```python
from build123d import *

# Parameters (mm, degrees)
SKETCH1_W           = 96
SKETCH1_H           = 24.5
BOSS_EXTRUDE1_DEPTH = 3
BOSS_EXTRUDE2_DEPTH = 57
FILLET1_R           = 2
FILLET2_R           = 3
CUT_EXTRUDE1_REACH  = 117.231
CUT_EXTRUDE2_REACH  = 116.303
SKETCH5_W           = 16
SKETCH5_H           = 12
SKETCH5_W_2         = 24
BOSS_EXTRUDE3_DEPTH = 9
SKETCH6_W           = 2.75
SKETCH6_H           = 4
CUT_EXTRUDE3_DEPTH  = 6
LPATTERN1_COUNT     = 4
LPATTERN1_PITCH     = 3.75
SKETCH7_W           = 2.75
SKETCH7_H           = 4
CUT_EXTRUDE4_DEPTH  = 6
LPATTERN2_COUNT     = 6
LPATTERN2_PITCH     = 3.75


with BuildPart() as part:
    # Sketch1 → Boss-Extrude1 (new body)
    with BuildSketch(Plane(origin=(0, 0, 0), x_dir=(1, 0, 0), z_dir=(0, 1, 0))):
        with Locations((48, 12.25)):
            Rectangle(SKETCH1_W, SKETCH1_H)
    extrude(amount=BOSS_EXTRUDE1_DEPTH)

    # Sketch2 → Boss-Extrude2 (add)
    with BuildSketch(Plane(origin=(0, 3, 0), x_dir=(1, 0, 0), z_dir=(0, 1, 0))):
        Polygon((0, 0), (96, 0), (96, 3), (89, 3), (89, 24.5), (7, 24.5), (7, 3), (0, 3), align=None)
    extrude(amount=BOSS_EXTRUDE2_DEPTH)

    # Fillet1
    fillet1_edges = [part.edges().sort_by_distance(p)[0] for p in [
        (89, 31.5, -24.5),
        (7, 31.5, -24.5),
        (48, 60, -24.5),
    ]]
    fillet(fillet1_edges, radius=FILLET1_R)

    # Fillet2
    fillet2_edges = [part.edges().sort_by_distance(p)[0] for p in [
        (0, 60, -1.5),
        (96, 60, -1.5),
        (0, 1.5, -24.5),
        (96, 1.5, -24.5),
    ]]
    fillet(fillet2_edges, radius=FILLET2_R)

    # Sketch3 → Cut-Extrude1 (cut, up to next)
    with BuildSketch(Plane(origin=(0, 0, -3), x_dir=(-1, 0, 0), z_dir=(0, 0, -1)), mode=Mode.PRIVATE) as cut_extrude1_sk1:
        with BuildLine():
            Line((-93, 45.5), (-96, 45.5))
            Line((-96, 45.5), (-96, 40.5))
            Line((-96, 40.5), (-93, 40.5))
            ThreePointArc((-93, 40.5), (-90.5, 43), (-93, 45.5))
        make_face()
    cut_extrude1_tool1 = extrude(cut_extrude1_sk1.sketch, amount=-CUT_EXTRUDE1_REACH, mode=Mode.PRIVATE) & part.part
    # Sketch3 → Cut-Extrude1 (cut, up to next)
    with BuildSketch(Plane(origin=(0, 0, -3), x_dir=(-1, 0, 0), z_dir=(0, 0, -1)), mode=Mode.PRIVATE) as cut_extrude1_sk2:
        with BuildLine():
            Line((-93, 25.5), (-96, 25.5))
            Line((-96, 25.5), (-96, 20.5))
            Line((-96, 20.5), (-93, 20.5))
            ThreePointArc((-93, 20.5), (-90.5, 23), (-93, 25.5))
        make_face()
    cut_extrude1_tool2 = extrude(cut_extrude1_sk2.sketch, amount=-CUT_EXTRUDE1_REACH, mode=Mode.PRIVATE) & part.part
    # Sketch3 → Cut-Extrude1 (cut, up to next)
    with BuildSketch(Plane(origin=(0, 0, -3), x_dir=(-1, 0, 0), z_dir=(0, 0, -1)), mode=Mode.PRIVATE) as cut_extrude1_sk3:
        with BuildLine():
            Line((-3, 25.5), (0, 25.5))
            Line((0, 25.5), (0, 20.5))
            Line((0, 20.5), (-3, 20.5))
            ThreePointArc((-3, 20.5), (-5.5, 23), (-3, 25.5))
        make_face()
    cut_extrude1_tool3 = extrude(cut_extrude1_sk3.sketch, amount=-CUT_EXTRUDE1_REACH, mode=Mode.PRIVATE) & part.part
    # Sketch3 → Cut-Extrude1 (cut, up to next)
    with BuildSketch(Plane(origin=(0, 0, -3), x_dir=(-1, 0, 0), z_dir=(0, 0, -1)), mode=Mode.PRIVATE) as cut_extrude1_sk4:
        with BuildLine():
            Line((-3, 45.5), (0, 45.5))
            Line((0, 45.5), (0, 40.5))
            Line((0, 40.5), (-3, 40.5))
            ThreePointArc((-3, 40.5), (-5.5, 43), (-3, 45.5))
        make_face()
    cut_extrude1_tool4 = extrude(cut_extrude1_sk4.sketch, amount=-CUT_EXTRUDE1_REACH, mode=Mode.PRIVATE) & part.part
    add(cut_extrude1_tool1.solids().sort_by_distance((93.486888, 43, -3))[0], mode=Mode.SUBTRACT)
    add(cut_extrude1_tool2.solids().sort_by_distance((93.486888, 23, -3))[0], mode=Mode.SUBTRACT)
    add(cut_extrude1_tool3.solids().sort_by_distance((2.513112, 23, -3))[0], mode=Mode.SUBTRACT)
    add(cut_extrude1_tool4.solids().sort_by_distance((2.513112, 43, -3))[0], mode=Mode.SUBTRACT)

    # Sketch4 → Cut-Extrude2 (cut, up to next)
    with BuildSketch(Plane(origin=(0, 3, 0), x_dir=(1, 0, 0), z_dir=(0, 1, 0)), mode=Mode.PRIVATE) as cut_extrude2_sk1:
        with BuildLine():
            Line((3, 16.5), (0, 16.5))
            Line((0, 16.5), (0, 11.5))
            Line((0, 11.5), (3, 11.5))
            ThreePointArc((3, 11.5), (5.5, 14), (3, 16.5))
        make_face()
    cut_extrude2_tool1 = extrude(cut_extrude2_sk1.sketch, amount=-CUT_EXTRUDE2_REACH, mode=Mode.PRIVATE) & part.part
    # Sketch4 → Cut-Extrude2 (cut, up to next)
    with BuildSketch(Plane(origin=(0, 3, 0), x_dir=(1, 0, 0), z_dir=(0, 1, 0)), mode=Mode.PRIVATE) as cut_extrude2_sk2:
        with BuildLine():
            Line((93, 11.5), (96, 11.5))
            Line((96, 11.5), (96, 16.5))
            Line((96, 16.5), (93, 16.5))
            ThreePointArc((93, 16.5), (90.5, 14), (93, 11.5))
        make_face()
    cut_extrude2_tool2 = extrude(cut_extrude2_sk2.sketch, amount=-CUT_EXTRUDE2_REACH, mode=Mode.PRIVATE) & part.part
    add(cut_extrude2_tool1.solids().sort_by_distance((2.513112, 3, -14))[0], mode=Mode.SUBTRACT)
    add(cut_extrude2_tool2.solids().sort_by_distance((93.486888, 3, -14))[0], mode=Mode.SUBTRACT)

    # Sketch5 → Boss-Extrude3 (add)
    with BuildSketch(Plane(origin=(0, 60, 0), x_dir=(1, 0, 0), z_dir=(0, 1, 0))):
        with Locations((68.5, 12)):
            Rectangle(SKETCH5_W, SKETCH5_H)
        with Locations((27.5, 12)):
            Rectangle(SKETCH5_W_2, SKETCH5_H)
    extrude(amount=BOSS_EXTRUDE3_DEPTH)

    # Sketch6 → Cut-Extrude3 (cut)
    with BuildSketch(Plane(origin=(0, 69, 0), x_dir=(1, 0, 0), z_dir=(0, 1, 0))):
        with Locations((74.125, 9)):
            Rectangle(SKETCH6_W, SKETCH6_H)
    cut_extrude3 = extrude(amount=-CUT_EXTRUDE3_DEPTH, mode=Mode.SUBTRACT)

    # LPattern1: Cut-Extrude3 ×4
    with Locations(*[(-i * LPATTERN1_PITCH, 0, 0) for i in range(1, LPATTERN1_COUNT)]):
        add(cut_extrude3, mode=Mode.SUBTRACT)

    # Sketch7 → Cut-Extrude4 (cut)
    with BuildSketch(Plane(origin=(0, 69, 0), x_dir=(1, 0, 0), z_dir=(0, 1, 0))):
        with Locations((37.125, 9)):
            Rectangle(SKETCH7_W, SKETCH7_H)
    cut_extrude4 = extrude(amount=-CUT_EXTRUDE4_DEPTH, mode=Mode.SUBTRACT)

    # LPattern2: Cut-Extrude4 ×6
    with Locations(*[(-i * LPATTERN2_PITCH, 0, 0) for i in range(1, LPATTERN2_COUNT)]):
        add(cut_extrude4, mode=Mode.SUBTRACT)


solid = part.part
```
Source: CAD feature listing. Evaluate the final solid. Frame: model axes, mm. A direction names the side the tool comes from. Give positions to 0.01 mm unless a question says otherwise; leave off trailing zeros. Write each loop counter-clockwise with the first axis right and the second up, starting at its lowest first coordinate (ties: lowest second). Pieces come first, ordered by that corner, then holes.
1. First-contact query: pin 1 (1.2 mm diameter, centred on y = 65.5, z = -9.5, fed in from -X); pin 2 (2 mm diameter, centred on x = 66.5, z = -8.5, fed in from +Y); pin 3 (5 mm diameter, centred on x = 79.5, z = -14, fed in from +Y); pin 4 (12 mm diameter, centred on x = 71.5, z = -8, fed in from +Y). Flat tips, straight axial feed; report the tip coordinate or a pass-through.
2. Section query C-C (x = 42). Return the cut outline in (y, z).
3. Access query for faces 1 (the face through (30, 63, -9)), 2 (the face through (68, 64, -6)), 3 (the face through (7.6, 31.9, -23.93)), 4 (the face through (1, 20.5, -2)). Directions: +Z, -Z, +X, -X, +Y, -Y. A direction counts if a zero-diameter tool reaches every point of the face in a straight line with its end or side. Return the directions, or none.
4. Section query A-A (y = 61). Return the cut outline in (x, z), then the cut area to 3 significant figures.
5. Section query D-D (y = 23). Return the cut outline in (x, z), then the cut area to 3 significant figures.
6. Material intervals for line 1 along X through (y, z) = (23, -8.25); line 2 along Y through (x, z) = (51, -8); line 3 along Y through (x, z) = (19.5, -9.5), sorted ascending.
7. Section query B-B (z = -14). Return the cut outline in (x, y), then the cut area to 3 significant figures.
8. Pull-direction query (X, two-part tool) for faces 5 (the face through (31, 66, -9)), 6 (the face through (7, 31, -13)), 7 (the face through (96, 1, -19)); classes: +X half, -X half, draft (parallel to the pull), parting line (faces both ways), or undercut.
Output values:
1. pin 1: stops at x = 15.5
1. pin 2: stops at y = 63
1. pin 3: stops at y = 60
1. pin 4: stops at y = 69
2. outline: (0, -24.5) - (58, -24.5) arc R2 ccw to (60, -22.5) - (60, 0) - (0, 0) - close
3. face 1: +Y
3. face 2: +Z, +X, -X, +Y
3. face 3: -Z, -X, +Y
3. face 4: +Z, -Z, -X
4. outline: (15.5, -18) - (39.5, -18) - (39.5, -6) - (15.5, -6) - close; (60.5, -18) - (76.5, -18) - (76.5, -6) - (60.5, -6) - close
4. area: 480 mm2
5. outline: (5.5, -3) - (7, -3) - (7, -22.5) arc R2 ccw to (9, -24.5) - (87, -24.5) arc R2 ccw to (89, -22.5) - (89, -3) - (90.5, -3) - (90.5, 0) - (5.5, 0) - close
5. area: 2,020 mm2
6. line 1: x = 7 to 89
6. line 2: y = 0 to 60
6. line 3: y = 0 to 63
7. outline: (5.5, 0) - (90.5, 0) - (90.5, 3) - (89, 3) - (89, 60) - (76.5, 60) - (76.5, 69) - (60.5, 69) - (60.5, 60) - (39.5, 60) - (39.5, 69) - (15.5, 69) - (15.5, 60) - (7, 60) - (7, 3) - (5.5, 3) - close
7. area: 5,290 mm2
8. face 5: undercut
8. face 6: -X half
8. face 7: +X half
